Here's how the part is built. I have some questions about the finished solid (model axes, mm). Face numbers are marked on the shaded views. A direction names the side the tool comes from. Round coordinates to 2 decimals unless told otherwise and drop trailing zeros. Loops run counter-clockwise (first coordinate to the right, second up) from the corner with the lowest first, then second, coordinate; pieces in that order, holes last. Notation, with made-up numbers: M -8.5,-22 L 36.5,-22 A19 cw 36.5,-1 Z; hole C 24.25,-34 d11. An arc over 180 degrees is marked long. Write each question's results on one line, items separated by ' | '. Start each with the question number.
```python
from build123d import *

# Parameters (mm, degrees)
SKETCH1_R           = 3.57
BOSS_EXTRUDE1_DEPTH = 5


with BuildPart() as part:
    # Sketch1 → Boss-Extrude1 (new body)
    with BuildSketch(Plane(origin=(0, 0, 0), x_dir=(0, 0, -1), z_dir=(1, 0, 0))):
        with BuildLine():
            ThreePointArc((4.27020031, 4.313964454), (-21.36, 14.853878163), (-46.99020031, 4.313964454))
            ThreePointArc((-46.99020031, 4.313964454), (-45.212525236, -5.534638014), (-36.65944536, -0.338492916))
            ThreePointArc((-36.65944536, -0.338492916), (-34.472469129, 5.364814131), (-29.3762145, 8.732122411))
            ThreePointArc((-29.3762145, 8.732122411), (-21.056615852, 9.761945239), (-12.805336851, 8.281184769))
            ThreePointArc((-12.805336851, 8.281184769), (-8.116246419, 4.932321146), (-6.05344864, -0.447950405))
            ThreePointArc((-6.05344864, -0.447950405), (2.54243032, -5.511891514), (4.27020031, 4.313964454))
        make_face()
        Circle(SKETCH1_R, mode=Mode.SUBTRACT)
        with Locations((-42.72, 0)):
            Circle(SKETCH1_R, mode=Mode.SUBTRACT)
    extrude(amount=BOSS_EXTRUDE1_DEPTH)


solid = part.part
```
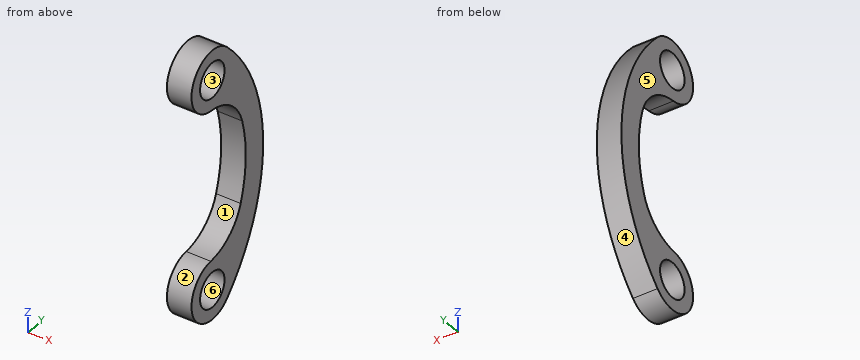
1. For pin 1 (4.5 mm diameter, centred on y = 0, z = 42.72, fed in from +X); pin 2 (2 mm diameter, centred on x = 1.5, z = 32.5, fed in from +Y); pin 3 (3 mm diameter, centred on x = 4, z = 2, fed in from +Y); pin 4 (1 mm diameter, centred on x = 4.5, z = 26.5, fed in from +Y), each with a flat end and sliding along its axis, tell me the tip position at first contact or that it passes through.
2. I want a section at D-D on z = 19.5. List the corners of the cut face in (x, y) for me, plus the area to 3 significant figures.
3. I need wall thicknesses on line 1 along Z through (x, y) = (1, -2.5); line 2 along Z through (x, y) = (2.2, 7.5); line 3 along Y through (x, z) = (2.9, -2.5). Which ranges of each line are inside material? Lowest first, please.
4. If we mould it in two halves opening along Y, with no side actions, what happens to the marked faces 3, 4, 5 and 6? For each: released by +Y, released by -Y, zero draft, split by the parting line, or undercut.
5. Which directions (+Z, -Z, +X, -X, +Y, -Y) give clear straight access to the entire face, cutting with the end or side of a thin tool? Please do the marked faces 1 and 2.
6. I want a section at B-B on z = 0. List the corners of the cut face in (x, y) for me, plus the area to 3 significant figures.
7. I want a section at C-C on y = 6.25. List the corners of the cut face in (x, z) for me, plus the area to 3 significant figures.
8. I want a section at A-A on x = 2.7. Count the separate pieces of the cut face and the enclosed holes in it, plus the area to 3 significant figures.
Outcome:
1) pin 1: through | pin 2: y = 13.41 | pin 3: y = 10.18 | pin 4: y = 14.56
2) outline: M 0,9.68 L 5,9.68 L 5,14.81 L 0,14.81 Z | area: 25.7 mm2
3) line 1: -5.53 to -2.55, 2.55 to 5.53, 37.19 to 40.17, 45.27 to 48.25 | line 2: -0.59 to 11.07, 32.11 to 43.31 | line 3: -5.53 to -2.55, 2.55 to 5.95
4) face 3: undercut | face 4: released by +Y | face 5: zero draft | face 6: undercut
5) face 1: +X, -X, -Y | face 2: +X, -X
6) outline: M 0,-6.07 L 5,-6.07 L 5,-3.57 L 0,-3.57 Z; M 0,3.57 L 5,3.57 L 5,7.94 L 0,7.94 Z | area: 34.3 mm2
7) outline: M 0,-2.15 L 5,-2.15 L 5,9.34 L 0,9.34 Z; M 0,33.67 L 5,33.67 L 5,44.87 L 0,44.87 Z | area: 113 mm2
8) separate pieces: 1 | enclosed holes: 2 | area: 400 mm2
